from build123d import *

# Parameters (mm, degrees)
SKETCH006_W     = 65
SKETCH006_H     = 60
PAD003_DEPTH    = 10
POCKET004_DEPTH = 10.001
POCKET005_DEPTH = 6.43
SKETCH009_W     = 1.05
SKETCH009_H     = 8.7
POCKET006_DEPTH = 15
SKETCH010_W     = 20
SKETCH010_H     = 26.8
POCKET007_DEPTH = 8.7
SKETCH011_W     = 2
SKETCH011_H     = 1.05
POCKET008_DEPTH = 8.7
SKETCH012_R     = 2
POCKET009_DEPTH = 10.001
CHAMFER_SIZE    = 1
CHAMFER001_SIZE = 1
CHAMFER002_SIZE = 2
FILLET002_R     = 1


with BuildPart() as part:
    # Sketch006 → Pad003 (new body)
    with BuildSketch(Plane.XY):
        Rectangle(SKETCH006_W, SKETCH006_H)
    extrude(amount=PAD003_DEPTH)

    # Sketch007 → Pocket004 (cut, through all)
    with BuildSketch(Plane.XY):
        Polygon((-19.3, 30), (-19.3, -15.8), (-14.8, -15.8), (-14.8, 1.8), (14.8, 1.8), (14.8, -15.8), (19.3, -15.8), (19.3, 30), align=None)
    extrude(amount=POCKET004_DEPTH, mode=Mode.SUBTRACT)

    # Sketch008 → Pocket005 (cut)
    with BuildSketch(Plane.XY):
        Polygon((-23.45, 30), (23.45, 30), (23.45, -15.8), (14.8, -15.8), (14.8, 1.8), (-14.8, 1.8), (-14.8, -15.8), (-23.45, -15.8), align=None)
    extrude(amount=POCKET005_DEPTH, mode=Mode.SUBTRACT)

    # Sketch009 (on DatumPlane) → Pocket006 (cut)
    with BuildSketch(Plane.XZ.offset(-1.8)):
        with Locations((-12, 4.35)):
            Rectangle(SKETCH009_W, SKETCH009_H)
        with Locations((12, 4.35)):
            Rectangle(SKETCH009_W, SKETCH009_H)
    extrude(amount=POCKET006_DEPTH, mode=Mode.SUBTRACT)

    # Sketch010 → Pocket007 (cut)
    with BuildSketch(Plane.XY):
        with Locations((0, -14.4)):
            Rectangle(SKETCH010_W, SKETCH010_H)
    extrude(amount=POCKET007_DEPTH, mode=Mode.SUBTRACT)

    # Sketch011 → Pocket008 (cut)
    with BuildSketch(Plane.XY):
        with Locations((-11, -3.525)):
            Rectangle(SKETCH011_W, SKETCH011_H)
        with Locations((11, -3.525)):
            Rectangle(SKETCH011_W, SKETCH011_H)
    extrude(amount=POCKET008_DEPTH, mode=Mode.SUBTRACT)

    # Sketch012 → Pocket009 (cut, through all)
    with BuildSketch(Plane.XY):
        with Locations((-27.975, 23)):
            Circle(SKETCH012_R)
        with Locations((27.975, 23)):
            Circle(SKETCH012_R)
        with Locations((27.975, -23)):
            Circle(SKETCH012_R)
        with Locations((-27.975, -23)):
            Circle(SKETCH012_R)
    extrude(amount=POCKET009_DEPTH, mode=Mode.SUBTRACT)

    # Chamfer
    chamfer_edges = [part.edges().sort_by_distance(p)[0] for p in [
        (19.3, 30, 8.215),
        (-19.3, 30, 8.215),
    ]]
    chamfer(chamfer_edges, length=CHAMFER_SIZE)

    # Chamfer001
    chamfer001_edges = [part.edges().sort_by_distance(p)[0] for p in [
        (14.8, 1.8, 8.215),
        (14.8, 1.8, 3.215),
        (-14.8, 1.8, 3.215),
        (-14.8, 1.8, 8.215),
    ]]
    chamfer(chamfer001_edges, length=CHAMFER001_SIZE)

    # Chamfer002
    chamfer002_edges = [part.edges().sort_by_distance(p)[0] for p in [
        (23.45, 30, 3.215),
        (-23.45, 30, 3.215),
    ]]
    chamfer(chamfer002_edges, length=CHAMFER002_SIZE)

    # Fillet002
    fillet002_edges = [part.edges().sort_by_distance(p)[0] for p in [
        (32.5, -30, 5),
        (-32.5, -30, 5),
    ]]
    fillet(fillet002_edges, radius=FILLET002_R)


solid = part.part
Verification items for the finished model (mm, model axes). A direction names the side the tool comes from. Give positions to 0.01 mm unless a question says otherwise; leave off trailing zeros. Loops run counter-clockwise (first coordinate to the right, second up) from the corner with the lowest first, then second, coordinate; pieces in that order, holes last.
1) Sectioned sample at C-C, the plane x = -8.5. Enter the section's corners in (y, z), then the cut area to 3 significant figures.
2) Sectioned sample at D-D, the plane z = 3.25. Count the separate pieces of the cut face and the enclosed holes in it, then the cut area to 3 significant figures.
3) Set-up check for faces 3 (the flat face through (-11.475, -9, 4)), 4 (the flat face through (0, -27.8, 4)), 5 (the flat face through (-28, 30, 6)), 6 (the flat face through (0, 1.8, 5)): record each of +Z, -Z, +X, -X, +Y, -Y from which the full face is reachable in a straight line by a thin tool's end or side.
4) Sectioned sample at A-A, the plane y = 19. Enter the section's corners in (x, z), then the cut area to 3 significant figures.
5) Sectioned sample at B-B, the plane y = -23. Enter the section's corners in (x, z) (3 decimals), then the cut area to 3 significant figures.
6) Thickness scan on line 1 along X through (y, z) = (-6.5, 4.25) (3 decimals); line 2 along X through (y, z) = (-9.5, 8) (3 decimals); line 3 along X through (y, z) = (-23, 7.5) (3 decimals). Record the ranges inside material, lowest first.
7) Draft check along X on faces 1 (the flat face through (10, -16, 4)), 2 (the flat face through (0, -6, 10)). Enter one of: pulls with the +X half, pulls with the -X half, needs draft (parallel to the pull), parting line crosses it, or undercut.
8) Depth check by flat-ended pin: pin 1 Ø1.5 at (x, z) = (1.5, 7.5) entering from +Y; pin 2 Ø4 at (x, z) = (18, 2) entering from +Y. Enter the tip coordinate at first touch or a pass-through.
Answers:
1. outline: (-30, 0) - (-27.8, 0) - (-27.8, 8.7) - (-1, 8.7) - (-1, 0) - (1.8, 0) - (1.8, 10) - (-30, 10) - close
1. area: 84.8 mm2
2. separate pieces: 2
2. enclosed holes: 4
2. area: 1,650 mm2
3. face 3: -Z, +Y
3. face 4: -Z
3. face 5: +Z, -Z, +X, -X, +Y
3. face 6: +Z, -Z, +Y
4. outline: (-32.5, 0) - (-23.45, 0) - (-23.45, 6.43) - (-19.3, 6.43) - (-19.3, 10) - (-32.5, 10) - close; (19.3, 6.43) - (23.45, 6.43) - (23.45, 0) - (32.5, 0) - (32.5, 10) - (19.3, 10) - close
4. area: 211 mm2
5. outline: (-32.5, 0) - (-29.975, 0) - (-29.975, 10) - (-32.5, 10) - close; (-25.975, 0) - (-10, 0) - (-10, 8.7) - (10, 8.7) - (10, 0) - (25.975, 0) - (25.975, 10) - (-25.975, 10) - close; (29.975, 0) - (32.5, 0) - (32.5, 10) - (29.975, 10) - close
5. area: 396 mm2
6. line 1: x = -32.5 to -23.45, -14.8 to -12.525, -11.475 to -10, 10 to 11.475, 12.525 to 14.8, 23.45 to 32.5
6. line 2: x = -32.5 to -19.3, -14.8 to -12.525, -11.475 to -10, 10 to 11.475, 12.525 to 14.8, 19.3 to 32.5
6. line 3: x = -32.5 to -29.975, -25.975 to -10, 10 to 25.975, 29.975 to 32.5
7. face 1: undercut
7. face 2: needs draft
8. pin 1: stops at y = 1.8
8. pin 2: stops at y = -15.8
